Part model, mm, in its own coordinate system. A direction names the side the tool comes from. Round coordinates to 2 decimals unless told otherwise and drop trailing zeros. Order: outer loops, then holes, each group sorted by start corner. A loop starts at its lowest first (then second) coordinate and runs counter-clockwise, first axis right, second up. Notation, with made-up numbers: M -15,80 L -4,80 A15 cw -4,102 Z; hole C 49,68 d1. An arc over 180 degrees is marked long. Write each question's results on one line, items separated by ' | '. Start each with the question number.
1. Band-saw the part on D-D, the plane y = -7. List the corners of the cut face in (x, z).
2. Which spindle directions (+Z, -Z, +X, -X, +Y, -Y) get a long thin tool onto all of the face, cutting with end or side? Do faces 1 (the face through (0, 7.6, 7)), 2 (the face through (9, 0, 16)), 3 (the face through (-6.92, -6.27, 17.74)). Say none if no direction does.
3. Band-saw the part on A-A, the plane z = 13.5. List the corners of the cut face in (x, y).
4. Band-saw the part on C-C, the plane z = 22. List the corners of the cut face in (x, y), then the cut area to 3 significant figures.
5. Drop a flat-ended pin along its axis: pin 1 Ø4 at (y, z) = (1, 27) entering from -X. Give the stop position or say it passes through.
6. Probe L1, parallel to Y at x = -1.5, z = 13.5; L2, parallel to Y at x = -5.75, z = 29.5. List the from-to ranges inside material, lowest first. Write a range as [from, to].
7. Two-plate mould, pull along Y, no slides. Class faces 4 (the face through (0, -9, 16)), 5 (the face through (-7.6, 0, 7)), 6 (the face through (0, 0, 33)): +Y half, -Y half, draft (parallel to the pull), parting line (faces both ways), or undercut.
8. Band-saw the part on B-B, the plane x = -6.5. List the corners of the cut face in (y, z), then the cut area to 3 significant figures.
```python
from build123d import *

# Parameters (mm, degrees)
F0_W      = 18
F0_H      = 18
F1_DEPTH  = 25
F1_FACE_W = 18
F1_FACE_H = 18
F2_DEPTH  = 8
F3_W      = 6.5
F3_H      = 13
F4_DEPTH  = 4.1
F5_W      = 15.2
F5_H      = 15.2
F6_DEPTH  = 15
F7_R      = 0.8


with BuildPart() as f1:
    # F0 (on Top) → F1 (new body)
    with BuildSketch(Plane.XY):
        Rectangle(F0_W, F0_H)
    extrude(amount=F1_DEPTH)

    # F1_face (on face) → F2 (join)
    with BuildSketch(Plane.XY.offset(25)):
        Rectangle(F1_FACE_W, F1_FACE_H)
    extrude(amount=F2_DEPTH)

    # F3 (on face) → F4 (cut)
    with BuildSketch(Plane(origin=(-9, 0, 0), x_dir=(0, -1, 0), z_dir=(-1, 0, 0))):
        with Locations((3.25, 24)):
            Rectangle(F3_W, F3_H)
        with Locations((-3.25, 24)):
            Rectangle(F3_W, F3_H)
    extrude(amount=-F4_DEPTH, mode=Mode.SUBTRACT)

    # F5 (on face) → F6 (cut)
    with BuildSketch(Plane(origin=(0, 0, 0), x_dir=(1, 0, 0), z_dir=(0, 0, -1))):
        Rectangle(F5_W, F5_H)
    extrude(amount=-F6_DEPTH, mode=Mode.SUBTRACT)

    # F7
    f7_edges = [f1.edges().sort_by_distance(p)[0] for p in [
        (-6.95, 6.5, 30.5),
        (-6.95, -6.5, 30.5),
        (-6.95, -6.5, 17.5),
        (-6.95, 6.5, 17.5),
    ]]
    fillet(f7_edges, radius=F7_R)


solid = f1.part
```
Solution:
1) outline: M -9,0 L -7.6,0 L -7.6,15 L 7.6,15 L 7.6,0 L 9,0 L 9,33 L -9,33 Z
2) face 1: -Z | face 2: +Z, -Z, +X, +Y, -Y | face 3: -X
3) outline: M -9,-9 L 9,-9 L 9,9 L -9,9 Z; hole M -7.6,-7.6 L 7.6,-7.6 L 7.6,7.6 L -7.6,7.6 Z
4) outline: M -9,-9 L 9,-9 L 9,9 L -9,9 L -9,6.5 L -4.9,6.5 L -4.9,-6.5 L -9,-6.5 Z | area: 271 mm^2
5) pin 1: x = -4.9
6) L1: [-9, -7.6], [7.6, 9] | L2: [-9, -6.5], [6.5, 9]
7) face 4: -Y half | face 5: undercut | face 6: draft
8) outline: M -9,0 L -7.6,0 L -7.6,15 L 7.6,15 L 7.6,0 L 9,0 L 9,33 L -9,33 Z; hole M -6.5,18.3 A0.8 ccw -5.7,17.5 L 5.7,17.5 A0.8 ccw 6.5,18.3 L 6.5,29.7 A0.8 ccw 5.7,30.5 L -5.7,30.5 A0.8 ccw -6.5,29.7 Z | area: 198 mm^2
